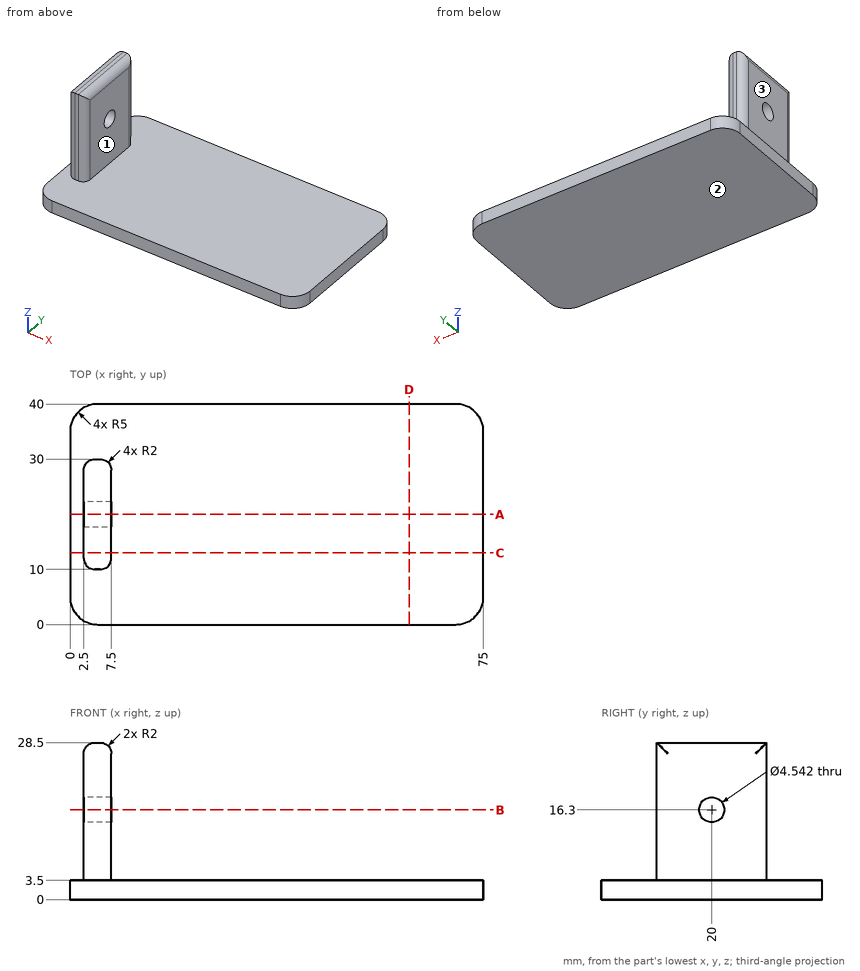
Check sheet for the drawn part. Datum: minimum x, y, z corner. Units: mm. A direction names the side the tool comes from. Round coordinates to 2 decimals unless told otherwise and drop trailing zeros. Order: outer loops, then holes, each group sorted by start corner. A loop starts at its lowest first (then second) coordinate and runs counter-clockwise, first axis right, second up.
(1) Cross-section at C-C, the plane y = 13. Enter the section's corners in (x, z), and give its area (3 significant figures).
(2) Cross-section at B-B, the plane z = 16.3. Enter the section's corners in (x, y).
(3) Access from +Z, -Z, +X, -X, +Y, -Y to the whole of each face (thin tool, end or side, straight path). Record for the marked faces 1, 2 and 3.
(4) Go/stop test with flat-tipped pins: P1, Ø0.8, axis at x = 5, z = 17, coming from the +Y side; P2, Ø3, axis at y = 25, z = 23.5, coming from the -X side; P3, Ø1.5, axis at y = 30.5, z = 9.5, coming from the +X side. Record where each tip stops, or that it passes through.
(5) Cross-section at A-A, the plane y = 20. Enter the section's corners in (x, z), and give its area (3 significant figures).
(6) Scan lines: probe 1 along Z at (x, y) = (4.45, 20); probe 2 along Z at (x, y) = (71, 33.5); probe 3 along X at (y, z) = (12.5, 20). Record each from-to range of solid material in increasing order.
(7) Cross-section at D-D, the plane x = 61.5. Enter the section's corners in (y, z), and give its area (3 significant figures).
Check sheet entries:
1. outline: (0, 0) - (75, 0) - (75, 3.5) - (7.5, 3.5) - (7.5, 26.5) arc R2 ccw to (5.5, 28.5) - (4.5, 28.5) arc R2 ccw to (2.5, 26.5) - (2.5, 3.5) - (0, 3.5) - close
1. area: 386 mm2
2. outline: (2.5, 12) arc R2 ccw to (4.5, 10) - (5.5, 10) arc R2 ccw to (7.5, 12) - (7.5, 17.73) - (2.5, 17.73) - close; (2.5, 22.27) - (7.5, 22.27) - (7.5, 28) arc R2 ccw to (5.5, 30) - (4.5, 30) arc R2 ccw to (2.5, 28) - close
3. face 1: +Z, +X, +Y, -Y
3. face 2: -Z, +X, -X, +Y, -Y
3. face 3: +Z, -X, +Y, -Y
4. P1: stops at y = 30
4. P2: stops at x = 2.5
4. P3: stops at x = 6.47
5. outline: (0, 0) - (75, 0) - (75, 3.5) - (7.5, 3.5) - (7.5, 14.03) - (2.5, 14.03) - (2.5, 3.5) - (0, 3.5) - close; (2.5, 18.57) - (7.5, 18.57) - (7.5, 26.5) arc R2 ccw to (5.5, 28.5) - (4.5, 28.5) arc R2 ccw to (2.5, 26.5) - close
5. area: 363 mm2
6. probe 1: z = 0 to 14.03, 18.57 to 28.5
6. probe 2: z = 0 to 3.5
6. probe 3: x = 2.5 to 7.5
7. outline: (0, 0) - (40, 0) - (40, 3.5) - (0, 3.5) - close
7. area: 140 mm2
